Work out the finished part from the listing and answer in its coordinate system (mm). A direction names the side the tool comes from. Give positions to 0.01 mm unless a question says otherwise; leave off trailing zeros. Loops run counter-clockwise (first coordinate to the right, second up) from the corner with the lowest first, then second, coordinate; pieces in that order, holes last.
```python
from build123d import *

# Parameters (mm, degrees)
EXTRUDE_1_DEPTH     = 3
SKETCH_3_W          = 20
SKETCH_3_H          = 31.5
EXTRUDE_2_DEPTH     = 2
SKETCH_4_R          = 0.5
CUT_EXTRUDE_1_DEPTH = 10
SKETCH_5_R          = 1.6
CUT_EXTRUDE_2_DEPTH = 10
SKETCH_6_R          = 1.75
CUT_EXTRUDE_3_DEPTH = 17
CUT_EXTRUDE_4_DEPTH = 1.6
EXTRUDE_3_DEPTH     = 3
SKETCH_9_W          = 31.5
SKETCH_9_H          = 1.6
EXTRUDE_4_DEPTH     = 3
SKETCH_10_R         = 1.75
SKETCH_10_R_2       = 0.5
CUT_EXTRUDE_5_DEPTH = 10
SKETCH_12_R         = 10
EXTRUDE_6_DEPTH     = 1.6
SKETCH_13_W         = 31.5
SKETCH_13_H         = 1.6
EXTRUDE_7_DEPTH     = 2
SKETCH_15_R         = 1.75
SKETCH_15_R_2       = 0.5
CUT_EXTRUDE_6_DEPTH = 12


with BuildPart() as part:
    # 草图1 → 凸台-拉伸1 (new body)
    with BuildSketch(Plane(origin=(0, 0, 0), x_dir=(1, 0, 0), z_dir=(0, 1, 0))):
        with BuildLine():
            Line((0, -15.75), (55, -15.75))
            Line((55, -15.75), (55, 15.75))
            Line((55, 15.75), (0, 15.75))
            ThreePointArc((0, 15.75), (-15.75, 0), (0, -15.75))
        make_face()
    extrude(amount=EXTRUDE_1_DEPTH)

    # 草图3 → 凸台-拉伸2 (add)
    with BuildSketch(Plane.XZ):
        with Locations((45, 0)):
            Rectangle(SKETCH_3_W, SKETCH_3_H)
    extrude(amount=EXTRUDE_2_DEPTH)

    # 草图4 → 切除-拉伸1 (cut)
    with BuildSketch(Plane.XZ):
        with Locations((0, 7)):
            Circle(SKETCH_4_R)
        with Locations((7, 0)):
            Circle(SKETCH_4_R)
        with Locations((0, -7)):
            Circle(SKETCH_4_R)
        with Locations((-7, 0)):
            Circle(SKETCH_4_R)
    extrude(amount=-CUT_EXTRUDE_1_DEPTH, mode=Mode.SUBTRACT)

    # 草图5 → 切除-拉伸2 (cut)
    with BuildSketch(Plane.XZ.offset(2)):
        with Locations((45, -4.5)):
            Circle(SKETCH_5_R)
        with Locations((45, 4.5)):
            Circle(SKETCH_5_R)
    extrude(amount=-CUT_EXTRUDE_2_DEPTH, mode=Mode.SUBTRACT)

    # 草图6 → 切除-拉伸3 (cut)
    with BuildSketch(Plane.XZ):
        Circle(SKETCH_6_R)
    extrude(amount=-CUT_EXTRUDE_3_DEPTH, mode=Mode.SUBTRACT)

    # 草图7 → 切除-拉伸4 (cut)
    with BuildSketch(Plane.XZ):
        with BuildLine():
            Line((35, -15.75), (35, 15.75))
            Line((35, 15.75), (0, 15.75))
            ThreePointArc((0, 15.75), (-15.75, 0), (0, -15.75))
            Line((0, -15.75), (35, -15.75))
        make_face()
    extrude(amount=-CUT_EXTRUDE_4_DEPTH, mode=Mode.SUBTRACT)

    # 草图8 → 凸台-拉伸3 (add)
    with BuildSketch(Plane.XZ.offset(-1.6)):
        with BuildLine():
            Line((0, -15.75), (35, -15.75))
            Line((35, -15.75), (35, 15.75))
            Line((35, 15.75), (0, 15.75))
            ThreePointArc((0, 15.75), (-15.75, 0), (0, -15.75))
        make_face()
    extrude(amount=-EXTRUDE_3_DEPTH)

    # 草图9 → 凸台-拉伸4 (add)
    with BuildSketch(Plane(origin=(35, 0, 0), x_dir=(0, 0, -1), z_dir=(1, 0, 0))):
        with Locations((0, 3.8)):
            Rectangle(SKETCH_9_W, SKETCH_9_H)
    extrude(amount=EXTRUDE_4_DEPTH)

    # 草图10 → 切除-拉伸5 (cut)
    with BuildSketch(Plane.XZ.offset(-1.6)):
        Circle(SKETCH_10_R)
        with Locations((0, 7)):
            Circle(SKETCH_10_R_2)
        with Locations((7, 0)):
            Circle(SKETCH_10_R_2)
        with Locations((0, -7)):
            Circle(SKETCH_10_R_2)
        with Locations((-7, 0)):
            Circle(SKETCH_10_R_2)
    extrude(amount=-CUT_EXTRUDE_5_DEPTH, mode=Mode.SUBTRACT)

    # 草图12 → 凸台-拉伸6 (add)
    with BuildSketch(Plane.XZ.offset(-1.6)):
        Circle(SKETCH_12_R)
    extrude(amount=EXTRUDE_6_DEPTH)

    # 草图13 → 凸台-拉伸7 (add)
    with BuildSketch(Plane(origin=(38, 0, 0), x_dir=(0, 0, -1), z_dir=(1, 0, 0))):
        with Locations((0, 3.8)):
            Rectangle(SKETCH_13_W, SKETCH_13_H)
    extrude(amount=EXTRUDE_7_DEPTH)

    # 草图15 → 切除-拉伸6 (cut)
    with BuildSketch(Plane.XZ):
        Circle(SKETCH_15_R)
        with Locations((7, 0)):
            Circle(SKETCH_15_R_2)
        with Locations((0, -7)):
            Circle(SKETCH_15_R_2)
        with Locations((0, 7)):
            Circle(SKETCH_15_R_2)
        with Locations((-7, 0)):
            Circle(SKETCH_15_R_2)
    extrude(amount=-CUT_EXTRUDE_6_DEPTH, mode=Mode.SUBTRACT)


solid = part.part
```
Q1. Given pin 1 (1 mm diameter, centred on x = 9.5, z = -2.5, fed in from -Y); pin 2 (3 mm diameter, centred on y = -0.5, z = 5.5, fed in from -X); pin 3 (1.8 mm diameter, centred on y = 4, z = -5, fed in from +X), each flat-ended and moving along its own axis, determine where each tip first touches the part or whether it passes through.
Q2. Section C-C on z = -9 is taken. Give the vertices of the cut face in (x, y).
Q3. Section A-A on z = 13.5 is taken. Give the vertices of the cut face in (x, y), plus the area to 3 significant figures.
Q4. Section B-B on x = 14.5 is taken. Give the vertices of the cut face in (y, z), plus the area to 3 significant figures.
Q5. Determine the mould class of faces 5 (the face through (1.617, 2.268, -0.67)), 6 (the face through (-15.746, 3.079, -0.346)), 7 (the face through (12, 4.6, 0)) for opening direction Z: +Z half, -Z half, draft (parallel to the pull), parting line (faces both ways), or undercut.
Q6. Consider line 1 along Z through (x, y) = (0, 3.4); line 2 along Z through (x, y) = (45, 0.15); line 3 along Z through (x, y) = (0, 1.3). Determine where each line is inside the solid, lowest interval first.
Q7. Which of the six approach directions +Z, -Z, +X, -X, +Y, -Y give full straight-line access (tool end or side, diameter ignored) to faces 1 (the face through (0, 0, -2)), 2 (the face through (35, 0, 0)), 3 (the face through (15, 1.6, 0)), 4 (the face through (40, 4, 0))?
Check result:
1. pin 1: stops at y = 0
1. pin 2: stops at x = -9.13
1. pin 3: stops at x = 40
2. outline: (-12.93, 1.6) - (-4.36, 1.6) - (-4.36, 0) - (4.36, 0) - (4.36, 1.6) - (35, 1.6) - (35, -2) - (55, -2) - (55, 3) - (40, 3) - (40, 4.6) - (-12.93, 4.6) - close
3. outline: (-8.11, 1.6) - (35, 1.6) - (35, -2) - (55, -2) - (55, 3) - (40, 3) - (40, 4.6) - (-8.11, 4.6) - close
3. area: 237 mm2
4. outline: (1.6, -15.75) - (4.6, -15.75) - (4.6, 15.75) - (1.6, 15.75) - close
4. area: 94.5 mm2
5. face 5: undercut
5. face 6: parting line
5. face 7: draft
6. line 1: z = -15.75 to -7.5, -6.5 to -1.75, 1.75 to 6.5, 7.5 to 15.75
6. line 2: z = -15.75 to -6.1, -2.9 to 2.9, 6.1 to 15.75
6. line 3: z = -10 to -7.5, -6.5 to -1.75, 1.75 to 6.5, 7.5 to 10
7. face 1: +Z, -Z, -X, -Y
7. face 2: +Z, -Z, -Y
7. face 3: -Y
7. face 4: +Z, -Z, +X, +Y
